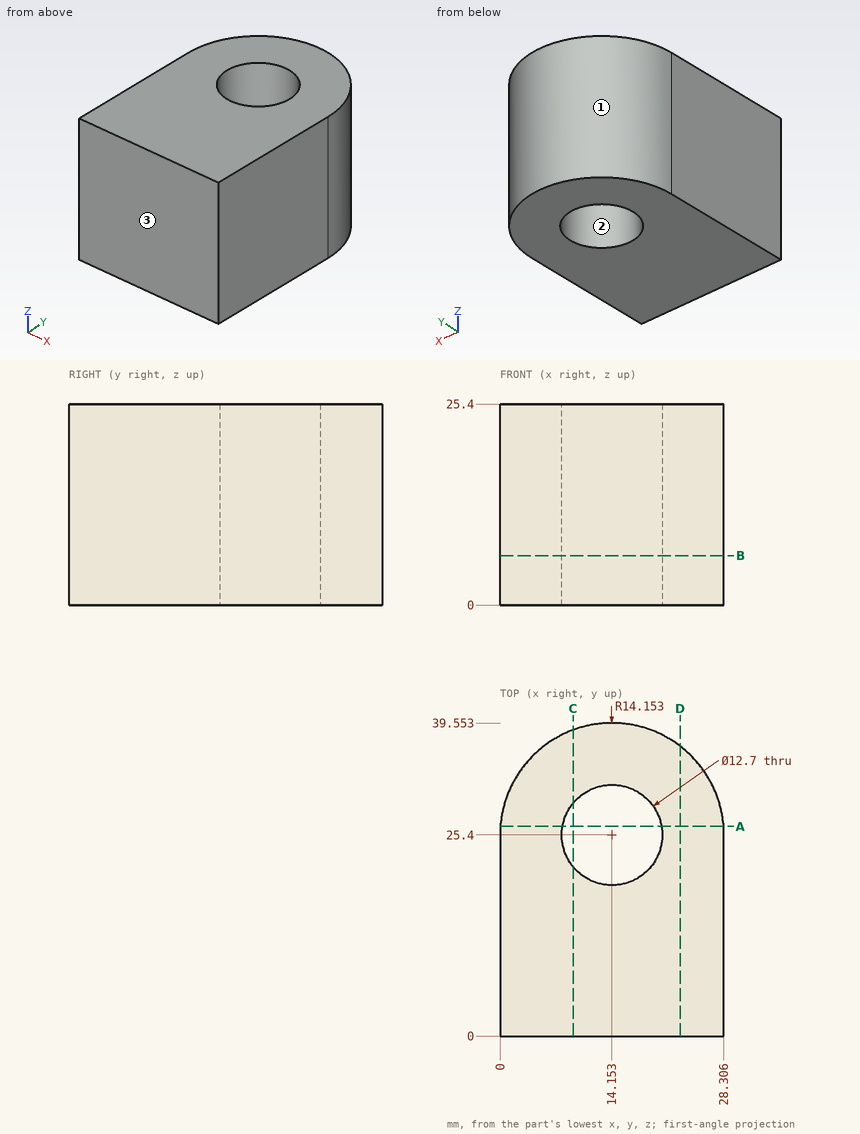
Study the drawing (mm; zero at the part's minimum x, y, z) and answer. Give positions to 0.01 mm unless a question says otherwise; leave off trailing zeros. Loops run counter-clockwise (first coordinate to the right, second up) from the corner with the lowest first, then second, coordinate; pieces in that order, holes last. Notation, with made-up numbers: (63, 29.5) -> (95, 29.5) arc R33 ccw to (95, 63.5) -> close; hole circle Ø3 at (52, 43.25). An arc over 180 degrees is marked (long way). Write item = value, one per line. Start each with the question number.
(1) The mould has two halves that part along Y. Classify the marked faces 1, 2 and 3: +Y half, -Y half, draft (parallel to the pull), parting line (faces both ways), or undercut.
(2) Given pin 1 Ø1.5 at (x, z) = (19.5, 22.5) entering from +Y (1 decimal); pin 2 Ø8 at (y, z) = (32.5, 21.5) entering from +X; pin 3 Ø4 at (y, z) = (35, 14) entering from +X, each flat-ended and moving along its own axis, determine where each tip first touches the part or whether it passes through.
(3) Find section B-B on z = 6.25. Give the vertices of the cut face in (x, y), and give its area (3 significant figures).
(4) Find the intervals of material crossed by probe 1 along X at (y, z) = (24.5, 12.5); probe 2 along X at (y, z) = (30, 7.5) (1 decimal); probe 3 along Y at (x, z) = (5, 4.5) (1 decimal), in increasing order. Write a range as from..to.
(5) Find section C-C on x = 9.25. Give the vertices of the cut face in (y, z) (1 decimal).
(6) Find section A-A on y = 26.5. Give the vertices of the cut face in (x, z), and give its area (3 significant figures).
(7) Find section D-D on x = 22.75. Give the vertices of the cut face in (y, z).
From the geometry:
q1.face_1 = +Y half
q1.face_2 = undercut
q1.face_3 = -Y half
q2.pin_1 = 38.8
q2.pin_2 = 27.96
q2.pin_3 = 26.09
q3.outline = (0, 0) -> (28.31, 0) -> (28.31, 25.4) arc R14.15 ccw to (0, 25.4) -> close; hole circle Ø12.7 at (14.15, 25.4)
q3.area = 907 mm^2
q4.probe_1 = 0..7.87, 20.44..28.31
q4.probe_2 = 0.8..9.8, 18.5..27.5
q4.probe_3 = 0..36.2
q5.outline = (0, 0) -> (21.4, 0) -> (21.4, 25.4) -> (0, 25.4) -> close; (29.4, 0) -> (38.7, 0) -> (38.7, 25.4) -> (29.4, 25.4) -> close
q6.outline = (0.04, 0) -> (7.9, 0) -> (7.9, 25.4) -> (0.04, 25.4) -> close; (20.41, 0) -> (28.26, 0) -> (28.26, 25.4) -> (20.41, 25.4) -> close
q6.area = 399 mm^2
q7.outline = (0, 0) -> (36.64, 0) -> (36.64, 25.4) -> (0, 25.4) -> close
